Verification items for the finished model (mm, model axes). Face numbers are marked on the shaded views. A direction names the side the tool comes from. Coordinates: 2 decimals unless noted, no trailing zeros. Write each loop counter-clockwise with the first axis right and the second up, starting at its lowest first coordinate (ties: lowest second). Pieces come first, ordered by that corner, then holes. Notation, with made-up numbers: (63.25, 59.5) -> (113.25, 59.5) arc R16 ccw to (113.25, 75.5) -> close; hole circle Ø8 at (22.25, -35.5). An arc over 180 degrees is marked (long way). Write item = value, one per line. Start each with the question number.
(1) Section check C-C (x = 1). Record the cut outline in (y, z) (3 decimals), plus the area to 3 significant figures.
(2) Section check B-B (z = 0). Record the cut outline in (x, y).
(3) Material ranges on probe 1 along Y at (x, z) = (0, 8.75); probe 2 along Z at (x, y) = (2.75, 3.5) (3 decimals); probe 3 along X at (y, z) = (4.5, 6.75), recorded low to high. Write a range as [from, to].
(4) Set-up check for the marked faces 1, 2 and 3: record each of +Z, -Z, +X, -X, +Y, -Y from which the full face is reachable in a straight line by a thin tool's end or side.
(5) Mould release check, pull along Z, two halves, no side actions. Record for the marked faces 4, 5 and 6: released by +Z, released by -Z, zero draft, split by the parting line, or undercut.
(6) Section check A-A (y = 4.25). State how many separate pieces and enclosed holes the cut face has, plus the area to 3 significant figures.
(7) Section check D-D (x = -4.5). Record the cut outline in (y, z) (3 decimals), plus the area to 3 significant figures.
(8) Gauge pin test, flat ends, axial feed: pin 1 Ø5 at (y, z) = (11, 1) entering from +X; pin 2 Ø4 at (y, z) = (9.5, 4.5) entering from -X; pin 3 Ø6 at (x, z) = (-2.5, 7.5) entering from +Y; pin 4 Ø3 at (y, z) = (6, 0) entering from +X. Record the tip position at first contact, or that the pin passes through.
Autodesk Fusion 360 part; units mm, degrees
sketch "Sketch1" plane through (0, 0, 0) normal (0, 1, 0) x (1, 0, 0)
  line L0 (-13.97, -9.525) -> (-13.97, 9.525)
  line L1 (-13.97, 9.525) -> (13.97, 9.525)
  line L2 (13.97, 9.525) -> (13.97, -9.525)
  line L3 (13.97, -9.525) -> (-13.97, 9.525) construction
  line L4 (-13.97, -9.525) -> (13.97, 9.525) construction
  line L5 (5.08, 9.525) -> (5.08, -9.525) construction
  line L6 (5.08, 0) -> (13.97, 0) construction
  arc A0 (5.08, -9.525) -> (5.08, 9.525) centre (4.4223, 0) ccw
  line L7 (-13.97, 9.525) -> (13.97, 9.525)
  arc A1 (5.08, -9.525) -> (5.08, 9.525) centre (4.4223, 0) ccw
  line L8 (13.97, -9.525) -> (-13.97, -9.525)
  line L9 (-13.97, -9.525) -> (-13.97, 9.525)
  line L10 (-12.446, 8.001) -> (5.08, 8.001)
  line L11 (5.08, -8.001) -> (-12.446, -8.001)
  line L12 (-12.446, -8.001) -> (-12.446, 8.001)
  line L13 (13.97, 0) -> (12.446, 0) construction
  arc A2 (5.08, -8.001) -> (5.08, 8.001) centre (4.4176, 0) ccw
  line L14 (-10.922, 8.001) -> (-10.922, -8.001)
  line L15 (-9.398, 8.001) -> (-9.398, -8.001)
  line L16 (2.794, 9.525) -> (2.794, 8.001)
  line L17 (2.794, -8.001) -> (2.794, -9.525)
  line L18 (-2.54, 9.525) -> (-2.54, 8.001)
  line L19 (-2.54, -8.001) -> (-2.54, -9.525)
  line L20 (-4.826, 9.525) -> (-4.826, 8.001)
  line L21 (-4.826, -8.001) -> (-4.826, -9.525)
  line L22 (5.08, 9.525) -> (5.08, 8.001)
  line L23 (5.08, -8.001) -> (5.08, -9.525)
  line L24 (5.08, 0.4445) -> (8.89, 0.4445)
  line L25 (8.89, 0.4445) -> (8.89, -0.4445)
  line L26 (8.89, -0.4445) -> (5.08, -0.4445)
  line L27 (5.08, -0.4445) -> (5.08, 0.4445)
  line L28 (5.08, 0) -> (6.985, 0) construction
  line L29 (7.4295, 1.905) -> (6.5405, 1.905)
  line L30 (6.5405, 1.905) -> (6.5405, -1.905)
  line L31 (6.5405, -1.905) -> (7.4295, -1.905)
  line L32 (7.4295, -1.905) -> (7.4295, 1.905)
  line L33 (7.4295, 1.905) -> (6.5405, -1.905) construction
  line L34 (6.5405, 1.905) -> (7.4295, -1.905) construction
  point P0 (6.985, 0)
  dimension "d2" = 19.05
  dimension "d4" = 9.525
  dimension "d5" = 9.525
  dimension "d6" = 27.94
  dimension "d7" = 19.05
  dimension "d12" = 1.524
  dimension "d13" = 1.524
  dimension "d14" = 1.524
  dimension "d17" = 19.05
  dimension "d18" = 19.05
  dimension "d19" = 1.524
  dimension "d20" = 1.524
  dimension "d21" = 1.524
  dimension "d22" = 16.764
  dimension "d23" = 11.43
  dimension "d24" = 16.764
  dimension "d25" = 11.43
  dimension "d26" = 2.286
  dimension "d27" = 2.286
  dimension "d38" = 3.81
  dimension "d39" = 0.889
  dimension "d40" = 0.4445
  dimension "d41" = 1.905
  dimension "d42" = 0.889
  dimension "d43" = 3.81
extrude "Extrude1" add sketch "Sketch1" along normal blind 6.731 contours L0 L1 L7 L8 L9 L10 L11 L12 L20 L21 | A0 A1 A2 L22 L23 makes body 1 at (9.3779, 4.4873, -8.1609) makes body 2 at (-13.97, 4.4873, 3.175)
extrude "Extrude2" add sketch "Sketch1" along normal blind 12.192 contours L10 L11 L14 L15 bodies 2
extrude "Extrude3" add sketch "Sketch1" along normal blind 1.524 contours L10 L11 A2 L15 | L10 L11 L12 L14 | L24 L26 L27 L30 | L24 L29 L30 L32 | L24 L26 L30 L32 | L24 L25 L26 L32 | L26 L30 L31 L32 bodies 1 2
extrude "Extrude4" add sketch "Sketch1" along normal blind 2.54 contours L8 L11 L19 L21 | L1 L7 L10 L18 L20 | L8 L11 L17 L23 | L1 L7 L10 L16 L22 bodies 1
extrude "Extrude5" add sketch "Sketch1" along normal blind 6.35 contours L8 L11 L17 L19 | L1 L7 L10 L16 L18 bodies 1
extrude "Extrude6" add sketch "Sketch1" along normal blind 3.81 contours L24 L26 L27 L30 | L24 L29 L30 L32 | L24 L26 L30 L32 | L24 L25 L26 L32 | L26 L30 L31 L32 bodies 1
sketch "Sketch2" plane through (-10.922, 0, 0) normal (-1, 0, 0) x (0, 0, 1)
  line L0 (-8.001, 1.524) -> (8.001, 1.524)
  line L1 (8.001, 1.524) -> (8.001, 6.731)
  line L2 (8.001, 6.731) -> (8.001, 12.192)
  line L3 (8.001, 12.192) -> (-8.001, 12.192)
  line L4 (-8.001, 12.192) -> (-8.001, 6.731)
  line L5 (-8.001, 6.731) -> (-8.001, 1.524)
  line L6 (0, 12.192) -> (0, 10.668)
  arc A0 (-8.001, 12.192) -> (8.001, 12.192) centre (0, 32.4326) ccw
  dimension "d46" = 1.524
extrude "Extrude7" cut sketch "Sketch2" against normal up to surface (1.524 mm away) contours L3 L6 A0 | L3 L6 A0 bodies 1
sketch "Sketch3" plane through (0, 0, -9.525) normal (0, 0, -1) x (-1, 0, 0)
  line L0 (-5.08, 0) -> (13.97, 0)
  line L1 (13.97, 0) -> (13.97, 6.731)
  line L2 (13.97, 6.731) -> (4.826, 6.731)
  line L3 (4.826, 6.731) -> (4.826, 2.54)
  line L4 (4.826, 2.54) -> (2.54, 2.54)
  line L5 (2.54, 2.54) -> (2.54, 6.35)
  line L6 (2.54, 6.35) -> (-2.794, 6.35)
  line L7 (-2.794, 6.35) -> (-2.794, 2.54)
  line L8 (-2.794, 2.54) -> (-5.08, 2.54)
  line L9 (-5.08, 2.54) -> (-5.08, 0)
  line L10 (-2.794, 3.556) -> (2.54, 3.556) construction
  line L11 (-0.127, 6.35) -> (-0.127, 3.556) construction
  circle A0 centre (-0.127, 3.556) radius 1.524
  dimension "d49" = 2.667
  dimension "d50" = 2.794
  dimension "d51" = 3.048
extrude "Extrude8" cut sketch "Sketch3" against normal up to surface (19.05 mm away) contours A0 bodies 1
fillet "Fillet1" radius 0.508 12 edges at (-4.826, 6.731, -8.763) (-2.54, 6.35, -8.763) (2.794, 6.35, -8.763) (5.08, 6.731, -8.763) (5.08, 6.731, 8.763) (2.794, 6.35, 8.763) (-2.54, 6.35, 8.763) (-4.826, 6.731, 8.763) (5.08, 3.81, 0) (6.985, 3.81, -1.905) (6.985, 3.81, 1.905) (8.89, 3.81, 0) on bodies 1
ref_plane "WorkPlane2" through (5.08, 3.3655, 0) normal (-1, 0, 0) x (0, 0, 1)
sketch "Sketch6" plane through (5.08, 3.3655, 0) normal (-1, 0, 0) x (0, 0, -1)
  line L0 (9.524, -3.3789) -> (-9.526, -3.3789)
  arc A0 (9.524, -3.3789) -> (-9.526, -3.3789) centre (-0.001, -23.9778) ccw
  dimension "d58" = 19.05
extrude "Extrude9" cut sketch "Sketch6" against normal blind 8.89 bodies 1
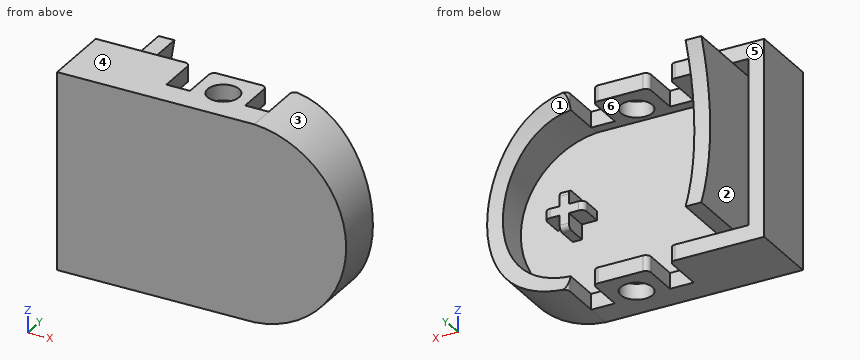
Response:
q1.outline = (0, -9.525) -> (2.307, -9.525) -> (2.307, -8.001) -> (1.524, -8.001) -> (1.524, 8.001) -> (2.307, 8.001) -> (2.307, 9.525) -> (0, 9.525) -> close; (4.805, -9.525) -> (6.35, -9.525) -> (6.35, -8.001) -> (4.805, -8.001) -> close; (4.805, 8.001) -> (6.35, 8.001) -> (6.35, 9.525) -> (4.805, 9.525) -> close
q1.area = 36.1 mm2
q2.outline = (-13.97, 0) -> (13.97, 0) -> (13.97, 4.65) -> (12.45, 4.65) -> (12.45, 1.52) -> (8.89, 1.52) -> (8.89, 3.3) arc R0.51 ccw to (8.38, 3.81) -> (5.59, 3.81) arc R0.51 ccw to (5.08, 3.3) -> (5.08, 1.52) -> (-9.4, 1.52) -> (-9.4, 10.67) -> (-10.92, 10.67) -> (-10.92, 1.52) -> (-12.45, 1.52) -> (-12.45, 6.73) -> (-13.97, 6.73) -> close
q3.probe_1 = [0, 2.04], [5.07, 6.35]
q3.probe_2 = [-9.525, -8.001], [8.001, 9.525]
q3.probe_3 = [-13.97, -12.45], [-10.92, -9.4], [8.76, 11.17]
q4.face_1 = +X, +Y
q4.face_2 = +Y
q4.face_3 = +X, +Y, -Y
q5.face_4 = released by +Z
q5.face_5 = zero draft
q5.face_6 = undercut
q6.separate_pieces = 6
q6.enclosed_holes = 1
q6.area = 125 mm2
q7.outline = (0, -9.525) -> (2.54, -9.525) -> (2.54, -8.001) -> (1.524, -8.001) -> (1.524, 8.001) -> (2.54, 8.001) -> (2.54, 9.525) -> (0, 9.525) -> close
q7.area = 32.1 mm2
q8.pin_1 = -9.4
q8.pin_2 = -10.92
q8.pin_3 = 6.73
q8.pin_4 = 13.97
